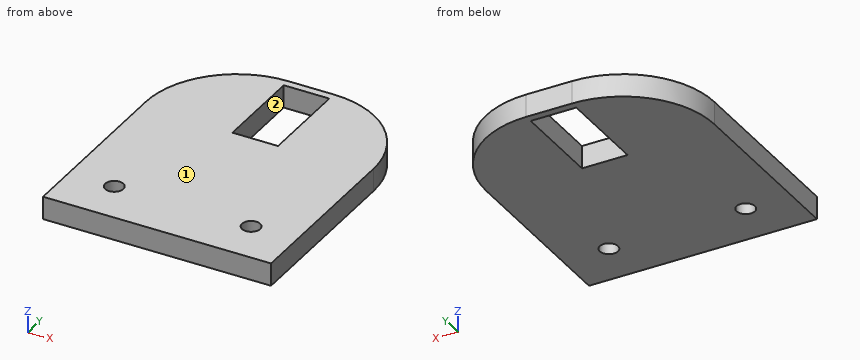
```python
from build123d import *

# Parameters (mm, degrees)
SKETCH1_W           = 50
SKETCH1_H           = 5
BOSS_EXTRUDE1_DEPTH = 60
FILLET1_R           = 20
SKETCH2_R           = 2
SKETCH2_W           = 10
SKETCH2_H           = 20
CUT_EXTRUDE1_DEPTH  = 5


with BuildPart() as part:
    # Sketch1 → Boss-Extrude1 (new body)
    with BuildSketch(Plane(origin=(0, 0, 0), x_dir=(1, 0, 0), z_dir=(0, 1, 0))):
        Rectangle(SKETCH1_W, SKETCH1_H)
    extrude(amount=BOSS_EXTRUDE1_DEPTH)

    # Fillet1
    fillet1_edges = [part.edges().sort_by_distance(p)[0] for p in [
        (25, 60, 0),
        (-25, 60, 0),
    ]]
    fillet(fillet1_edges, radius=FILLET1_R)

    # Sketch2 → Cut-Extrude1 (cut)
    with BuildSketch(Plane.XY.offset(2.5)):
        with Locations((-15, 10)):
            Circle(SKETCH2_R)
        with Locations((15, 10)):
            Circle(SKETCH2_R)
        with Locations((0, 48.271414018)):
            Rectangle(SKETCH2_W, SKETCH2_H)
    extrude(amount=-CUT_EXTRUDE1_DEPTH, mode=Mode.SUBTRACT)


solid = part.part
```
The model under review builds one solid part; all positions refer to its coordinate system, in mm. Face numbers are marked on the shaded views. A direction names the side the tool comes from. Round coordinates to 2 decimals unless told otherwise and drop trailing zeros. Write each loop counter-clockwise with the first axis right and the second up, starting at its lowest first coordinate (ties: lowest second). Pieces come first, ordered by that corner, then holes.
(1) We need section B-B on y = 10. Give the boundary of the cut face in (x, z).
(2) Machinability: for the marked faces 1 and 2, which of the approach directions +Z, -Z, +X, -X, +Y, -Y give a long, thin tool a straight path to every point of the face, cutting with its end or side? Answer none if there is none.
(3) We need section A-A on y = 56. Give the boundary of the cut face in (x, z).
(4) Insertion check: pin 1 (2.5 mm diameter, centred on x = -0.5, z = -0.5, fed in from -Y). The pin has a flat end and moves straight along its axis. Give the tip position at first contact, or say it passes through.
(5) We need section D-D on z = 1.05. Give the boundary of the cut face in (x, y).
(6) Wall thickness on L1, parallel to Y at x = -0.5, z = -1.6; L2, parallel to X at y = 39, z = -1.55; L3, parallel to X at y = 9, z = 2.2: over which ranges is each line inside the solid? List them lowest first.
(7) We need section C-C on x = -4. Give the boundary of the cut face in (y, z).
Findings below:
1. outline: (-25, -2.5) - (-17, -2.5) - (-17, 2.5) - (-25, 2.5) - close; (-13, -2.5) - (13, -2.5) - (13, 2.5) - (-13, 2.5) - close; (17, -2.5) - (25, -2.5) - (25, 2.5) - (17, 2.5) - close
2. face 1: +Z, +X, -X, +Y, -Y
2. face 2: +Z, -Z
3. outline: (-17, -2.5) - (-5, -2.5) - (-5, 2.5) - (-17, 2.5) - close; (5, -2.5) - (17, -2.5) - (17, 2.5) - (5, 2.5) - close
4. pin 1: stops at y = 0
5. outline: (-25, 0) - (25, 0) - (25, 40) arc R20 ccw to (5, 60) - (-5, 60) arc R20 ccw to (-25, 40) - close; hole circle Ø4 at (-15, 10); hole (-5, 38.27) - (5, 38.27) - (5, 58.27) - (-5, 58.27) - close; hole circle Ø4 at (15, 10)
6. L1: y = 0 to 38.27, 58.27 to 60
6. L2: x = -25 to -5, 5 to 25
6. L3: x = -25 to -16.73, -13.27 to 13.27, 16.73 to 25
7. outline: (0, -2.5) - (38.27, -2.5) - (38.27, 2.5) - (0, 2.5) - close; (58.27, -2.5) - (60, -2.5) - (60, 2.5) - (58.27, 2.5) - close
